The listing builds one solid part. Answer for the finished solid, in the listing's coordinates (mm). A direction names the side the tool comes from. Give positions to 0.01 mm unless a question says otherwise; leave off trailing zeros. Write each loop counter-clockwise with the first axis right and the second up, starting at its lowest first coordinate (ties: lowest second). Pieces come first, ordered by that corner, then holes. Notation, with made-up numbers: (23, -1) -> (65, -1) arc R18 cw to (65, 19) -> close; hole circle Ø9 at (-22, -3.75). An arc over 180 degrees is marked (long way). One line per question, with ' | ' between items.
from build123d import *

# Parameters (mm, degrees)
SKETCH1_W                 = 3
SKETCH1_H                 = 2.15
SKETCH1_W_2               = 8.2
SKETCH1_H_2               = 6.05
BODY_DEPTH                = 2.7
PINS_DEPTH                = 0.3
PINS_DEPTH_BACK           = 0.3
SKETCH2_W                 = 1.3
SKETCH2_H                 = 3.1
SKETCH3_R                 = 0.8
M1_6HOLES_DEPTH           = 12.906720791
FREEPOSITION_DEPTH        = 0.4
FREEPOSITION_DEPTH_BACK   = 0.4
OPERATINGPOINT_DEPTH      = 0.4
OPERATINGPOINT_DEPTH_BACK = 0.4


with BuildPart() as part:
    # Sketch1 → Body (new body)
    with BuildSketch(Plane(origin=(0, 0, 0), x_dir=(1, 0, 0), z_dir=(0, 1, 0))):
        with Locations((1.5, 7.125)):
            Rectangle(SKETCH1_W, SKETCH1_H)
        with Locations((4.1, 3.025)):
            Rectangle(SKETCH1_W_2, SKETCH1_H_2)
    extrude(amount=BODY_DEPTH)

    # Sketch2 → Pins (add, two sides: drawn at the far end of the back side and taken through both)
    with BuildSketch(Plane(origin=(0, 1.35, 0), x_dir=(1, 0, 0), z_dir=(0, 1, 0)).offset(-PINS_DEPTH_BACK)):
        with Locations((1.6, -1.55)):
            Rectangle(SKETCH2_W, SKETCH2_H)
        with Locations((4.1, -1.55)):
            Rectangle(SKETCH2_W, SKETCH2_H)
        with Locations((6.6, -1.55)):
            Rectangle(SKETCH2_W, SKETCH2_H)
    extrude(amount=PINS_DEPTH + PINS_DEPTH_BACK)

    # Sketch3 → M1.6Holes (cut, through all)
    with BuildSketch(Plane(origin=(0, 2.7, 0), x_dir=(1, 0, 0), z_dir=(0, 1, 0))):
        with Locations(Location((2.1, 1.6, 0), (0, 0, 270))):
            Circle(SKETCH3_R)
        with Locations(Location((6.1, 1.6, 0), (0, 0, 270))):
            Circle(SKETCH3_R)
    extrude(amount=-M1_6HOLES_DEPTH, mode=Mode.SUBTRACT)

    # Sketch4 → FreePosition (add, two sides: drawn at the far end of the back side and taken through both)
    with BuildSketch(Plane(origin=(0, 1.35, 0), x_dir=(1, 0, 0), z_dir=(0, 1, 0)).offset(-FREEPOSITION_DEPTH_BACK)):
        with BuildLine():
            ThreePointArc((7.115151319, 9.8), (7.022559042, 9.510139779), (6.779075529, 9.32763483))
            Line((6.779075529, 9.32763483), (7.251440659, 9.491558958))
            Line((7.251440659, 9.491558958), (7.08751651, 9.963924149))
            ThreePointArc((7.08751651, 9.963924149), (7.108194216, 9.883118604), (7.115151319, 9.8))
        make_face()
        with BuildLine():
            ThreePointArc((6.142786129, 9.636075851), (6.146132258, 9.626733962), (6.149663119, 9.617460317))
            Line((6.149663119, 9.617460317), (6.615151319, 9.8))
            Line((6.615151319, 9.8), (6.142786129, 9.636075851))
        make_face()
        with BuildLine():
            Line((6.615151319, 9.8), (6.149663119, 9.617460317))
            ThreePointArc((6.149663119, 9.617460317), (6.40602238, 9.345835837), (6.779075529, 9.32763483))
            ThreePointArc((6.779075529, 9.32763483), (7.022559042, 9.510139779), (7.115151319, 9.8))
            ThreePointArc((7.115151319, 9.8), (7.108194216, 9.883118604), (7.08751651, 9.963924149))
            ThreePointArc((7.08751651, 9.963924149), (6.45122717, 10.272365191), (6.142786129, 9.636075851))
            Line((6.142786129, 9.636075851), (6.615151319, 9.8))
        make_face()
        with BuildLine():
            Line((6.149663119, 9.617460317), (0.75, 7.5))
            Line((0.75, 7.5), (0.75, 7.235374235))
            Line((0.75, 7.235374235), (6.779075529, 9.32763483))
            ThreePointArc((6.779075529, 9.32763483), (6.40602238, 9.345835837), (6.149663119, 9.617460317))
        make_face()
        with BuildLine():
            Line((0.75, 7.764625765), (0.75, 7.5))
            Line((0.75, 7.5), (6.149663119, 9.617460317))
            ThreePointArc((6.149663119, 9.617460317), (6.146132258, 9.626733962), (6.142786129, 9.636075851))
            Line((6.142786129, 9.636075851), (0.75, 7.764625765))
        make_face()
    extrude(amount=FREEPOSITION_DEPTH + FREEPOSITION_DEPTH_BACK)

    # Sketch5 → OperatingPoint (add, two sides: drawn at the far end of the back side and taken through both)
    with BuildSketch(Plane(origin=(0, 1.35, 0), x_dir=(1, 0, 0), z_dir=(0, 1, 0)).offset(-OPERATINGPOINT_DEPTH_BACK)):
        with BuildLine():
            Line((0.75, 7.764625765), (0.75, 7.235374235))
            Line((0.75, 7.235374235), (7.047885091, 7.701363081))
            ThreePointArc((7.047885091, 7.701363081), (6.6836512, 7.822046181), (6.51219484, 8.165314959))
            Line((6.51219484, 8.165314959), (0.75, 7.764625765))
        make_face()
        with BuildLine():
            ThreePointArc((7.510990337, 8.2), (7.377355849, 7.859740817), (7.047885091, 7.701363081))
            Line((7.047885091, 7.701363081), (7.544317529, 7.738094773))
            Line((7.544317529, 7.738094773), (7.509785834, 8.234685041))
            ThreePointArc((7.509785834, 8.234685041), (7.510689121, 8.217352975), (7.510990337, 8.2))
        make_face()
        with BuildLine():
            ThreePointArc((6.51219484, 8.165314959), (6.6836512, 7.822046181), (7.047885091, 7.701363081))
            ThreePointArc((7.047885091, 7.701363081), (7.377355849, 7.859740817), (7.510990337, 8.2))
            ThreePointArc((7.510990337, 8.2), (7.510689121, 8.217352975), (7.509785834, 8.234685041))
            Line((7.509785834, 8.234685041), (7.010990337, 8.2))
            Line((7.010990337, 8.2), (6.51219484, 8.165314959))
        make_face()
        with BuildLine():
            ThreePointArc((7.509785834, 8.234685041), (6.976305296, 8.698795497), (6.51219484, 8.165314959))
            Line((6.51219484, 8.165314959), (7.010990337, 8.2))
            Line((7.010990337, 8.2), (7.509785834, 8.234685041))
        make_face()
    extrude(amount=OPERATINGPOINT_DEPTH + OPERATINGPOINT_DEPTH_BACK)


solid = part.part
Item 1: Determine the mould class of faces 1 (the face through (4.103, 1.344, -8.928)), 2 (the face through (5.2, 1.75, -7.9)), 3 (the face through (4.781, 1.344, -8.045)) for opening direction X: pulls with the +X half, pulls with the -X half, needs draft (parallel to the pull), parting line crosses it, or undercut.
Answers below:
face 1: pulls with the -X half | face 2: needs draft | face 3: undercut
Item 2: A tool of negligible diameter and unlimited length cuts with its end or side. For faces 4 (the face through (7, 1.65, 2)), 5 (the face through (5.2, 0.95, -7.9)), 6 (the face through (6, 1, -6.05)), 7 (the face through (4, 2.7, -4)), 8 (the face through (4, 1.05, 2)), from which of +Z, -Z, +X, -X, +Y, -Y can it reach the whole face along a straight path? Write none if from no direction.
Answers below:
face 4: +Z, +X, -X, +Y | face 5: -Z, +X, -Y | face 6: +X, +Y, -Y | face 7: +Z, -Z, +X, -X, +Y | face 8: +Z, +X, -X, -Y
Item 3: Find section B-B (y = 1.2). Count the separate pieces of the cut face and the enclosed holes in it, then the cut area to 3 significant figures.
Answers below:
separate pieces: 1 | enclosed holes: 2 | area: 69.6 mm²
Item 4: Consider line 1 (X direction, y = 1.6, z = -1.6); line 2 (X direction, y = 1.3, z = 1.5); line 3 (Z direction, x = 4, y = 1.7). Determine where each line is inside the solid, lowest interval first. Write a range as [from, to].
Answers below:
line 1: [0, 1.3], [2.9, 5.3], [6.9, 8.2] | line 2: [0.95, 2.25], [3.45, 4.75], [5.95, 7.25] | line 3: [-8.89, -8.36], [-7.99, -7.48], [-6.05, 0]
Item 5: Flat-ended cylindrical pins translate along their axes: pin 1 (1.4 mm diameter, centred on x = 1, y = 0.5, fed in from -Z); pin 2 (1 mm diameter, centred on x = 1.5, z = 2, fed in from +Y); pin 3 (1.8 mm diameter, centred on x = 4, z = -9.5, fed in from +Y). Find the tip coordinate at first contact, or state that the pin passes through.
Answers below:
pin 1: z = -8.2 | pin 2: y = 1.65 | pin 3: y = 1.75
Item 6: Find section A-A (z = -1.6). Write down the section's boundary in (x, y).
Answers below:
outline: (0, 0) -> (1.3, 0) -> (1.3, 2.7) -> (0, 2.7) -> close; (2.9, 0) -> (5.3, 0) -> (5.3, 2.7) -> (2.9, 2.7) -> close; (6.9, 0) -> (8.2, 0) -> (8.2, 2.7) -> (6.9, 2.7) -> close
Item 7: Find section C-C (x = 2.75). Write down the section's boundary in (y, z), then the cut area to 3 significant figures.
Answers below:
outline: (0, -8.2) -> (0.95, -8.2) -> (0.95, -8.46) -> (1.75, -8.46) -> (1.75, -8.2) -> (2.7, -8.2) -> (2.7, -2.07) -> (0, -2.07) -> close; (0, -1.13) -> (2.7, -1.13) -> (2.7, 0) -> (0, 0) -> close | area: 19.8 mm²
Item 8: Find section D-D (y = 2.4). Write down the section's boundary in (x, z).
Answers below:
outline: (0, -8.2) -> (3, -8.2) -> (3, -6.05) -> (8.2, -6.05) -> (8.2, 0) -> (0, 0) -> close; hole circle Ø1.6 at (2.1, -1.6); hole circle Ø1.6 at (6.1, -1.6)
